```python
from build123d import *

# Parameters (mm, degrees)
F1_DEPTH      = 6.35
F2_R          = 19.05
F2_R_2        = 4.7625
F4_DEPTH      = 69.85
F3_R          = 12.7
F5_DEPTH      = 63.5
F5_DEPTH_BACK = 25.4
F6_R          = 5.08


with BuildPart() as f1:
    # F0 (on Top) → F1 (new body)
    with BuildSketch(Plane.XY):
        with BuildLine():
            Line((0, 9.398), (0, 0))
            Line((0, 0), (101.6, 0))
            Line((101.6, 0), (101.6, 9.398))
            Line((101.6, 9.398), (85.852, 9.398))
            ThreePointArc((85.852, 9.398), (76.2, 19.05), (85.852, 28.702))
            Line((85.852, 28.702), (101.6, 28.702))
            Line((101.6, 28.702), (101.6, 38.1))
            Line((101.6, 38.1), (0, 38.1))
            Line((0, 38.1), (0, 28.702))
            Line((0, 28.702), (15.748, 28.702))
            ThreePointArc((15.748, 28.702), (25.4, 19.05), (15.748, 9.398))
            Line((15.748, 9.398), (0, 9.398))
        make_face()
    extrude(amount=F1_DEPTH)

    # F2 (on Top) → F4 (join)
    with BuildSketch(Plane.XY):
        with Locations((50.8, 19.05)):
            Circle(F2_R)
        with Locations((50.8, 19.05)):
            Circle(F2_R_2, mode=Mode.SUBTRACT)
    extrude(amount=-F4_DEPTH)

    # F3 (on Top) → F5 (cut, two sides)
    with BuildSketch(Plane.XY) as f5_sk:
        with Locations((50.8, 19.05)):
            Circle(F3_R)
    extrude(amount=-F5_DEPTH, mode=Mode.SUBTRACT)
    extrude(f5_sk.sketch, amount=F5_DEPTH_BACK, mode=Mode.SUBTRACT)

    # F6
    f6_edges = [f1.edges().sort_by_distance(p)[0] for p in [
        (101.6, 0, 3.175),
        (101.6, 38.1, 3.175),
        (0, 0, 3.175),
        (0, 38.1, 3.175),
    ]]
    fillet(f6_edges, radius=F6_R)


solid = f1.part
```
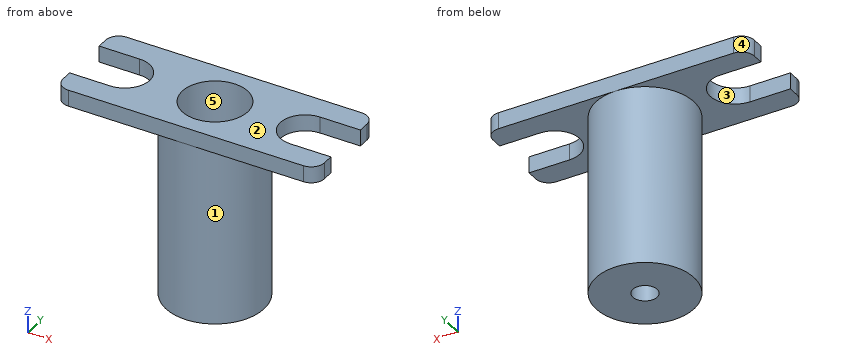
Source: CAD feature listing. Evaluate the final solid. Frame: model axes, mm. Face numbers are marked on the shaded views. A direction names the side the tool comes from. Round coordinates to 2 decimals unless told otherwise and drop trailing zeros. Loops run counter-clockwise (first coordinate to the right, second up) from the corner with the lowest first, then second, coordinate; pieces in that order, holes last.
(1) Section query A-A (y = 19.05). Output: boundary loops of the cut face in (x, z), and give its area (3 significant figures).
From the geometry:
outline: (25.4, 0) - (31.75, 0) - (31.75, -69.85) - (46.04, -69.85) - (46.04, -63.5) - (38.1, -63.5) - (38.1, 6.35) - (25.4, 6.35) - close; (55.56, -69.85) - (69.85, -69.85) - (69.85, 0) - (76.2, 0) - (76.2, 6.35) - (63.5, 6.35) - (63.5, -63.5) - (55.56, -63.5) - close
area: 1,150 mm2
(2) Section query B-B (x = 77.5). Output: boundary loops of the cut face in (y, z).
From the geometry:
outline: (0, 0) - (14.21, 0) - (14.21, 6.35) - (0, 6.35) - close; (23.89, 0) - (38.1, 0) - (38.1, 6.35) - (23.89, 6.35) - close
(3) Pull-direction query (Y, two-part tool) for the marked faces 1, 2 and 3; classes: +Y half, -Y half, draft (parallel to the pull), parting line (faces both ways), or undercut.
From the geometry:
face 1: parting line
face 2: draft
face 3: undercut
(4) Material intervals for probe 1 along X at (y, z) = (19.05, -26); probe 2 along Y at (x, z) = (50.8, -67); probe 3 along Z at (x, y) = (92.5, 4.5), sorted ascending.
From the geometry:
probe 1: x = 31.75 to 38.1, 63.5 to 69.85
probe 2: y = 0 to 14.29, 23.81 to 38.1
probe 3: z = 0 to 6.35
(5) Section query C-C (z = -13.5). Output: boundary loops of the cut face in (x, y), and give its area (3 significant figures).
From the geometry:
outline: circle Ø38.1 at (50.8, 19.05); hole circle Ø25.4 at (50.8, 19.05)
area: 633 mm2
(6) Section query D-D (y = 25). Output: boundary loops of the cut face in (x, z).
From the geometry:
outline: (23.35, 0) - (32.7, 0) - (32.7, -69.85) - (68.9, -69.85) - (68.9, 0) - (78.25, 0) - (78.25, 6.35) - (62.02, 6.35) - (62.02, -63.5) - (39.58, -63.5) - (39.58, 6.35) - (23.35, 6.35) - close
(7) Contact query for flat-ended pins moving along their axis: pin 1 Ø1.5 at (x, z) = (45, -34) entering from -Y; pin 2 Ø10 at (x, z) = (30, -29) entering from -Y; pin 3 Ø5 at (y, z) = (16.5, -61) entering from +X. Output: stop coordinate, or through.
From the geometry:
pin 1: stops at y = 0.68
pin 2: stops at y = 8.41
pin 3: stops at x = 69.85
(8) Access query for the marked faces 4 and 5. Directions: +Z, -Z, +X, -X, +Y, -Y. A direction counts if a zero-diameter tool reaches every point of the face in a straight line with its end or side. Return the directions, or none.
From the geometry:
face 4: +Z, -Z, -X, +Y
face 5: +Z
